```python
from build123d import *

# Parameters (mm, degrees)
F0_W     = 20
F0_H     = 20
F1_DEPTH = 2
F3_DEPTH = 18
F5_DEPTH = 18


with BuildPart() as f1:
    # F0 (on Top) → F1 (new body)
    with BuildSketch(Plane.XY):
        with Locations((4.142752, 7.774246)):
            Rectangle(F0_W, F0_H)
    extrude(amount=F1_DEPTH)

    # F2 (on face) → F3 (join)
    with BuildSketch(Plane.XY.offset(2)):
        Polygon((14.142752, 17.774246), (-5.857248, 17.774246), (-5.857248, 15.774246), (12.142752, 15.774246), (12.142752, -2.225754), (14.142752, -2.225754), align=None)
    extrude(amount=F3_DEPTH)

    # F4 (on face) → F5 (join)
    with BuildSketch(Plane.XY.offset(2)):
        Polygon((8.142752, 11.774246), (-5.857248, 11.774246), (-5.857248, 9.767495), (6.612573, 9.774246), (6.612573, -2.225754), (8.612573, -2.225754), (8.612573, 11.774246), align=None)
    extrude(amount=F5_DEPTH)


solid = f1.part
```
Geometry check sheet. Reference: the model listing, model coordinates, mm. A direction names the side the tool comes from. Give positions to 0.01 mm unless a question says otherwise; leave off trailing zeros. Write each loop counter-clockwise with the first axis right and the second up, starting at its lowest first coordinate (ties: lowest second). Pieces come first, ordered by that corner, then holes.
1) Section check C-C, the plane x = 7.75. Record the boundary of the cut face in (y, z), and give its area (3 significant figures).
2) Release check for a two-part mould opening along X. For faces 1 (the flat face through (12.143, 7, 11)), 2 (the flat face through (14.143, 8, 10)), 3 (the flat face through (8.613, 5, 11)), 4 (the flat face through (4, 8, 0)) record: pulls with the +X half, pulls with the -X half, needs draft (parallel to the pull), parting line crosses it, or undercut.
3) Gauge pin test, flat ends, axial feed: pin 1 (1 mm diameter, centred on x = -3, z = 3.5, fed in from -Y); pin 2 (4 mm diameter, centred on y = 3.5, z = 8, fed in from -X); pin 3 (1.5 mm diameter, centred on x = 1, y = 4, fed in from +Z). Record the tip position at first contact, or that the pin passes through.
4) Section check B-B, the plane y = 7.5. Record the boundary of the cut face in (x, z), and give its area (3 significant figures).
5) Section check A-A, the plane z = 6. Record the boundary of the cut face in (x, y).
6) Material ranges on L1, parallel to X at y = 3.25, z = 15.5; L2, parallel to Y at x = 4.25, z = 18.25; L3, parallel to Y at x = 8, z = 14.75, recorded low to high.
7) Access from +Z, -Z, +X, -X, +Y, -Y to the whole of each face (thin tool, end or side, straight path). Record for faces 5 (the flat face through (3, 15.774, 11)), 6 (the flat face through (6.613, 4, 11)), 7 (the flat face through (8, 16, 20)).
8) Section check D-D, the plane y = 14.25. Record the boundary of the cut face in (x, z), and give its area (3 significant figures).
Computed:
1. outline: (-2.23, 0) - (17.77, 0) - (17.77, 20) - (15.77, 20) - (15.77, 2) - (11.77, 2) - (11.77, 20) - (-2.23, 20) - close
1. area: 328 mm2
2. face 1: undercut
2. face 2: pulls with the +X half
2. face 3: undercut
2. face 4: needs draft
3. pin 1: stops at y = 9.77
3. pin 2: stops at x = 6.61
3. pin 3: stops at z = 2
4. outline: (-5.86, 0) - (14.14, 0) - (14.14, 20) - (12.14, 20) - (12.14, 2) - (8.61, 2) - (8.61, 20) - (6.61, 20) - (6.61, 2) - (-5.86, 2) - close
4. area: 112 mm2
5. outline: (-5.86, 9.77) - (6.61, 9.77) - (6.61, -2.23) - (8.61, -2.23) - (8.61, 11.77) - (-5.86, 11.77) - close; (-5.86, 15.77) - (12.14, 15.77) - (12.14, -2.23) - (14.14, -2.23) - (14.14, 17.77) - (-5.86, 17.77) - close
6. L1: x = 6.61 to 8.61, 12.14 to 14.14
6. L2: y = 9.77 to 11.77, 15.77 to 17.77
6. L3: y = -2.23 to 11.77, 15.77 to 17.77
7. face 5: +Z, -X
7. face 6: +Z, -X, -Y
7. face 7: +Z, +X, -X, +Y, -Y
8. outline: (-5.86, 0) - (14.14, 0) - (14.14, 20) - (12.14, 20) - (12.14, 2) - (-5.86, 2) - close
8. area: 76.0 mm2
